The listing builds one solid part. Answer for the finished solid, in the listing's coordinates (mm). A direction names the side the tool comes from. Coordinates: 2 decimals unless noted, no trailing zeros. Order: outer loops, then holes, each group sorted by start corner. A loop starts at its lowest first (then second) coordinate and runs counter-clockwise, first axis right, second up. Notation, with made-up numbers: (-9, 64.5) -> (44, 64.5) arc R25 ccw to (44, 92.5) -> close; hole circle Ø7 at (-38, 64.5). An arc over 180 degrees is marked (long way). Write item = value, one per line. Start each with the question number.
```python
from build123d import *

# Parameters (mm, degrees)
SKETCH1_W                        = 480.822
SKETCH1_H                        = 76.2
BASE_FLANGE1_DEPTH               = 2.032
EDGE_FLANGE3_START               = -240.411
EDGE_FLANGE3_DEPTH               = 480.822
EDGE_FLANGE3_2_DEPTH             = 480.822
EDGE_FLANGE1_DEPTH               = 70.328201504
EDGE_FLANGE1_BEND_DEPTH          = 70.328201504
EDGE_FLANGE2_DEPTH               = 480.822
F_11_32_0_34375_DIAMETER_HOLE1_D = 8.73125
F_17_64_0_26563_DIAMETER_HOLE1_D = 6.747002
FILLET1_R                        = 3.175
SKETCH25_W                       = 47.165600752
SKETCH25_H                       = 38.1
CUT_EXTRUDE1_DEPTH               = 655.776434505
EDGE_FLANGE4_DEPTH               = 480.822
FILLET2_R                        = 3.175


# Read off the part's stored shape, not the designer's step: Edge-Flange3
# Sheet-metal steps are written as plain solids
with BuildPart() as part:
    # Sketch1 → Base-Flange1 (new body)
    with BuildSketch(Plane(origin=(0, 0, 0), x_dir=(1, 0, 0), z_dir=(0, 1, 0))):
        Rectangle(SKETCH1_W, SKETCH1_H)
    extrude(amount=-BASE_FLANGE1_DEPTH)

    # Edge-Flange3 outline → Edge-Flange3 (cut)
    with BuildSketch(Plane.YZ.offset(EDGE_FLANGE3_START)):
        with BuildLine():
            ThreePointArc((-2.032, 32.228201504), (-1.958948217, 32.995292327), (-1.742419128, 33.734805713))
            Line((-1.742419128, 33.734805713), (0, 38.1))
            Line((0, 38.1), (-2.032, 38.1))
            Line((-2.032, 38.1), (-2.032, 32.228201504))
        make_face()
    extrude(amount=EDGE_FLANGE3_DEPTH, mode=Mode.SUBTRACT)

    # Edge-Flange3 2 outline → Edge-Flange3 2 (add)
    with BuildSketch(Plane.YZ.offset(EDGE_FLANGE3_START)):
        with BuildLine():
            Line((148.005784856, 408.891387665), (0, 38.1))
            Line((0, 38.1), (0, 32.228201504))
            ThreePointArc((0, 32.228201504), (0.036525892, 32.611746915), (0.144790436, 32.981503608))
            Line((0.144790436, 32.981503608), (149.89299442, 408.13808556))
            Line((149.89299442, 408.13808556), (148.005784856, 408.891387665))
        make_face()
    extrude(amount=EDGE_FLANGE3_2_DEPTH)

    # Edge-Flange1 section (across the edge) → Edge-Flange1 (add)
    with BuildSketch(Plane(origin=(-242.443, 0, -38.1), x_dir=(1, 0, 0), z_dir=(0, 0, 1))):
        with BuildLine():
            Line((-2.032, 2.032), (-2.032, 36.068))
            Line((-2.032, 36.068), (0, 36.068))
            Line((0, 36.068), (0, 2.032))
            ThreePointArc((0, 2.032), (0.595159021, 0.595159021), (2.032, 0))
            Line((2.032, 0), (2.032, -2.032))
            ThreePointArc((2.032, -2.032), (-0.841681959, -0.841681959), (-2.032, 2.032))
        make_face()
    extrude(amount=EDGE_FLANGE1_DEPTH)

    # Edge-Flange1 section 2 (across the edge) → Edge-Flange1 bend (add)
    with BuildSketch(Plane(origin=(242.443, 0, 32.228201504), x_dir=(-1, 0, 0), z_dir=(0, 0, -1))):
        with BuildLine():
            Line((-2.032, 2.032), (-2.032, 36.068))
            Line((-2.032, 36.068), (0, 36.068))
            Line((0, 36.068), (0, 2.032))
            ThreePointArc((0, 2.032), (0.595159021, 0.595159021), (2.032, 0))
            Line((2.032, 0), (2.032, -2.032))
            ThreePointArc((2.032, -2.032), (-0.841681959, -0.841681959), (-2.032, 2.032))
        make_face()
    extrude(amount=EDGE_FLANGE1_BEND_DEPTH)

    # Edge-Flange2 section (across the edge) → Edge-Flange2 (add)
    with BuildSketch(Plane(origin=(240.411, 0, -40.132), x_dir=(0, 0, 1), z_dir=(-1, 0, 0))):
        with BuildLine():
            Line((-2.032, 2.032), (-2.032, 36.068))
            Line((-2.032, 36.068), (0, 36.068))
            Line((0, 36.068), (0, 2.032))
            ThreePointArc((0, 2.032), (0.595159021, 0.595159021), (2.032, 0))
            Line((2.032, 0), (2.032, -2.032))
            ThreePointArc((2.032, -2.032), (-0.841681959, -0.841681959), (-2.032, 2.032))
        make_face()
    extrude(amount=EDGE_FLANGE2_DEPTH)

    # 11/32 (0.34375) Diameter Hole1 (through all)
    with Locations(Plane(origin=(244.475, 0, 0), x_dir=(0, 0, -1), z_dir=(1, 0, 0))):
        with Locations((-17.557349869, 19.03458979)):
            Hole(F_11_32_0_34375_DIAMETER_HOLE1_D / 2)

    # 17/64 (0.26563) Diameter Hole1 (through all)
    with Locations(Plane(origin=(0, -13.117977393, 5.236196428), x_dir=(-1, 0, 0), z_dir=(0, -0.9287448642521535, 0.370719539713311))):
        with Locations((225.425, -79.024412767), (225.425, -231.424412767), (225.425, -383.824412767), (-225.425, -383.824412767), (-225.425, -231.424412767), (-225.425, -79.024412767)):
            Hole(F_17_64_0_26563_DIAMETER_HOLE1_D / 2)

    # Fillet1
    fillet1_edges = [part.edges().sort_by_distance(p)[0] for p in [
        (-240.411, 148.949389638, 408.514736612),
        (240.411, 148.949389638, 408.514736612),
        (-243.459, 36.068, -38.1),
        (-243.459, 36.068, 32.228201504),
        (243.459, 36.068, 32.228201504),
        (243.459, 36.068, -38.1),
        (240.411, 36.068, -41.148),
        (-240.411, 36.068, -41.148),
    ]]
    fillet(fillet1_edges, radius=FILLET1_R)

    # Sketch25 → Cut-Extrude1 (cut, through all)
    with BuildSketch(Plane(origin=(244.475, 0, 0), x_dir=(0, 0, -1), z_dir=(1, 0, 0))):
        with Locations((18.581199624, 17.018)):
            Rectangle(SKETCH25_W, SKETCH25_H)
    extrude(amount=-CUT_EXTRUDE1_DEPTH, mode=Mode.SUBTRACT)

    # Edge-Flange4 section (across the edge) → Edge-Flange4 (add)
    with BuildSketch(Plane(origin=(240.411, 0, 4.010528132), x_dir=(0, 0.6156614753256621, 0.788010753606719), z_dir=(-1, 0, 0))):
        with BuildLine():
            Line((-2.032, 0.99107262), (-2.032, 50.8))
            Line((-2.032, 50.8), (0, 50.8))
            Line((0, 50.8), (0, 0.99107262))
            ThreePointArc((0, 0.99107262), (0.205650498, 0.10030245), (0.780975882, -0.610165231))
            Line((0.780975882, -0.610165231), (-0.470048236, -2.211403083))
            ThreePointArc((-0.470048236, -2.211403083), (-1.620699004, -0.790467721), (-2.032, 0.99107262))
        make_face()
    extrude(amount=EDGE_FLANGE4_DEPTH)

    # Fillet2
    fillet2_edges = [part.edges().sort_by_distance(p)[0] for p in [
        (-243.459, 36.068, 5.001600752),
        (243.459, 36.068, 5.001600752),
        (240.411, 39.405434224, -28.06569374),
        (-240.411, 39.405434224, -28.06569374),
    ]]
    fillet(fillet2_edges, radius=FILLET2_R)


solid = part.part
```
Item 1: Section A-A, the plane x = -126 is taken. Give the vertices of the cut face in (y, z), then the cut area to 3 significant figures.
Item 2: Consider probe 1 along Y at (x, z) = (-24, 30); probe 2 along Y at (x, z) = (159, 135.5). Determine where each line is inside the solid, lowest interval first.
Item 3: For a pull along Z with two mould halves and no side action, classify faces 4 (the flat face through (-3.37, 73.97, 217.93)), 5 (the flat face through (-3, 0, 18)), 6 (the flat face through (3.37, 18.88, -13.32)), 7 (the flat face through (240.411, 17, -11)) as pulls with the +Z half, pulls with the -Z half, needs draft (parallel to the pull), parting line crosses it, or undercut.
Item 4: Section B-B, the plane y = 48 is taken. Give the vertices of the cut face in (x, z), then the cut area to 3 significant figures.
Item 5: Each of these flat-tipped pins is pushed along its axis until it touches: pin 1 (2 mm diameter, centred on x = -242, y = 10.5, fed in from -Z); pin 2 (4 mm diameter, centred on x = 63.5, y = 27.5, fed in from -Z); pin 3 (22 mm diameter, centred on x = -29.5, z = 14, fed in from +Y). Where does it stop, or does it pass through?
Item 6: Which of the six approach directions +Z, -Z, +X, -X, +Y, -Y give full straight-line access (tool end or side, diameter ignored) to faces 1 (the flat face through (3.366, 20.681, -12.147)), 2 (the flat face through (242.443, 23, 22)), 3 (the flat face through (-244.475, 15, 21))?
Item 7: Section C-C, the plane z = 230 is taken. Give the vertices of the cut face in (x, y).
A:
q1.outline = (-2.03, 5) arc R4.06 ccw to (-0.47, 1.8) -> (38.78, -28.87) -> (40.03, -27.27) -> (0.78, 3.4) arc R2.03 cw to (0, 5) -> (0, 32.23) arc R2.03 cw to (0.14, 32.98) -> (149.89, 408.14) -> (148.01, 408.89) -> (-1.74, 33.73) arc R4.06 ccw to (-2.03, 32.23) -> close
q1.area = 985 mm^2
q2.probe_1 = -2.03 to 0
q2.probe_2 = 38.88 to 41.07
q3.face_4 = undercut
q3.face_5 = undercut
q3.face_6 = pulls with the -Z half
q3.face_7 = needs draft
q4.outline = (-240.41, 152.87) -> (240.41, 152.87) -> (240.41, 158.35) -> (-240.41, 158.35) -> close
q4.area = 2,640 mm^2
q5.pin_1 = 5
q5.pin_2 = -21.62
q5.pin_3 = 1.29
q6.face_1 = +X, -X, +Y
q6.face_2 = +Z, -Z, +Y
q6.face_3 = +Z, -Z, -X, +Y, -Y
q7.outline = (-240.41, 76.6) -> (240.41, 76.6) -> (240.41, 78.79) -> (-240.41, 78.79) -> close
